Could you check a few things on this drawing? It's one solid part, dimensions in mm from its lowest x, y, z. A direction names the side the tool comes from. Give positions to 0.01 mm unless a question says otherwise; leave off trailing zeros. Loops run counter-clockwise (first coordinate to the right, second up) from the corner with the lowest first, then second, coordinate; pieces in that order, holes last. Notation, with made-up numbers: (58, -40) -> (77, -40) arc R22 cw to (77, -4) -> close; hole circle Ø2 at (58.5, 64). An arc over 180 degrees is marked (long way). One line per question, with ' | ' between items.
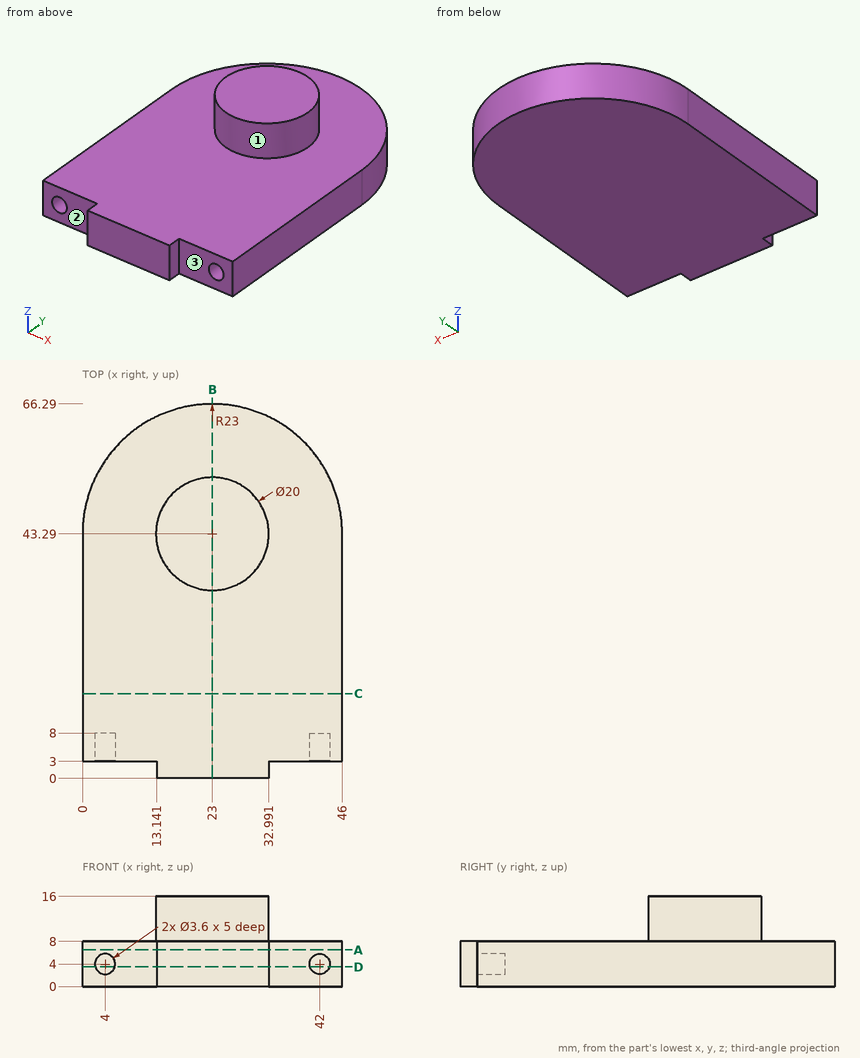
Q1. If we section it at A-A (z = 6.5): Write out the boundary of the cut face in (x, y), plus the area to 3 significant figures.
Entries:
outline: (0, 3) -> (13.14, 3) -> (13.14, 0) -> (32.99, 0) -> (32.99, 3) -> (46, 3) -> (46, 43.29) arc R23 ccw to (0, 43.29) -> close | area: 2,740 mm²
Q2. If we section it at D-D (z = 3.5): Write out the boundary of the cut face in (x, y), plus the area to 3 significant figures.
Entries:
outline: (0, 3) -> (2.27, 3) -> (2.27, 8) -> (5.73, 8) -> (5.73, 3) -> (13.14, 3) -> (13.14, 0) -> (32.99, 0) -> (32.99, 3) -> (40.27, 3) -> (40.27, 8) -> (43.73, 8) -> (43.73, 3) -> (46, 3) -> (46, 43.29) arc R23 ccw to (0, 43.29) -> close | area: 2,710 mm²
Q3. If I drill on probe 1 along X at (y, z) = (4.75, 4); probe 2 along Z at (x, y) = (42, 6.9); probe 3 along Z at (x, y) = (33.5, 7.5), over which ranges is the centre line in solid material (lowest first)? Write a range as from..to.
Entries:
probe 1: 0..2.2, 5.8..40.2, 43.8..46 | probe 2: 0..2.2, 5.8..8 | probe 3: 0..8
Q4. If we section it at B-B (x = 23): Write out the boundary of the cut face in (y, z), plus the area to 3 significant figures.
Entries:
outline: (0, 0) -> (66.29, 0) -> (66.29, 8) -> (53.29, 8) -> (53.29, 16) -> (33.29, 16) -> (33.29, 8) -> (0, 8) -> close | area: 690 mm²
Q5. On a 3-axis mill with a long thin cutter (end or side, diameter ignored), from which of +Z, -Z, +X, -X, +Y, -Y can I reach the whole of each face in a straight line? I mean the marked faces 1, 2 and 3. Say none if no direction works.
Entries:
face 1: +Z | face 2: +Z, -Z, -X, -Y | face 3: +Z, -Z, +X, -Y
Q6. If we section it at C-C (y = 15): Write out the boundary of the cut face in (x, z).
Entries:
outline: (0, 0) -> (46, 0) -> (46, 8) -> (0, 8) -> close
Q7. For pin 1 Ø0.9 at (y, z) = (1.5, 4.5) entering from -X; pin 2 Ø6.5 at (x, z) = (8.5, 5.5) entering from -Y; pin 3 Ø1 at (x, z) = (21.5, 3) entering from +Y, each with a flat end and sliding along its axis, tell me the tip position at first contact or that it passes through.
Entries:
pin 1: x = 13.14 | pin 2: y = 3 | pin 3: y = 66.27
